Drawing for the job (mm, zero at the part's lowest x, y, z). A direction names the side the tool comes from. Coordinates: 2 decimals unless noted, no trailing zeros. Write each loop counter-clockwise with the first axis right and the second up, starting at its lowest first coordinate (ties: lowest second). Pieces come first, ordered by that corner, then holes. Notation, with made-up numbers: M 53,-9.75 L 58,-9.75 A19 ccw 58,-0.75 Z; hole C 1.5,88 d7. An arc over 180 degrees is marked long. Use a Markdown table: item, result. Add a question column.
Q1. Slice it at C-C on x = 11. Write the cut outline in (y, z), then the cut area to 3 significant figures.
Q2. Slice it at B-B on z = 1.5. Write the cut outline in (x, y).
Q3. Pin check, flat tips, straight feed: pin 1 Ø1.5 at (x, z) = (7, 7.5) entering from -Y; pin 2 Ø4 at (y, z) = (18, 4.5) entering from -X; pin 3 Ø1 at (x, y) = (1.5, 25.5) entering from -Z; pin 4 Ø3 at (x, y) = (8, 43) entering from +Z. Stop position of each tip, or through.
Q4. Wall check: L1, parallel to Y at x = 11.5, z = 4.5; L2, parallel to X at y = 19.5, z = 4.75 (1 decimal); L3, parallel to Z at x = 6.75, y = 6 (1 decimal). Give the ranges that are in metal, low to high. Write a range as from..to.
Q5. Tool access for the marked faces 1 and 2: list every direction of +Z, -Z, +X, -X, +Y, -Y with a clear straight run to the whole face (end or side of a thin tool).
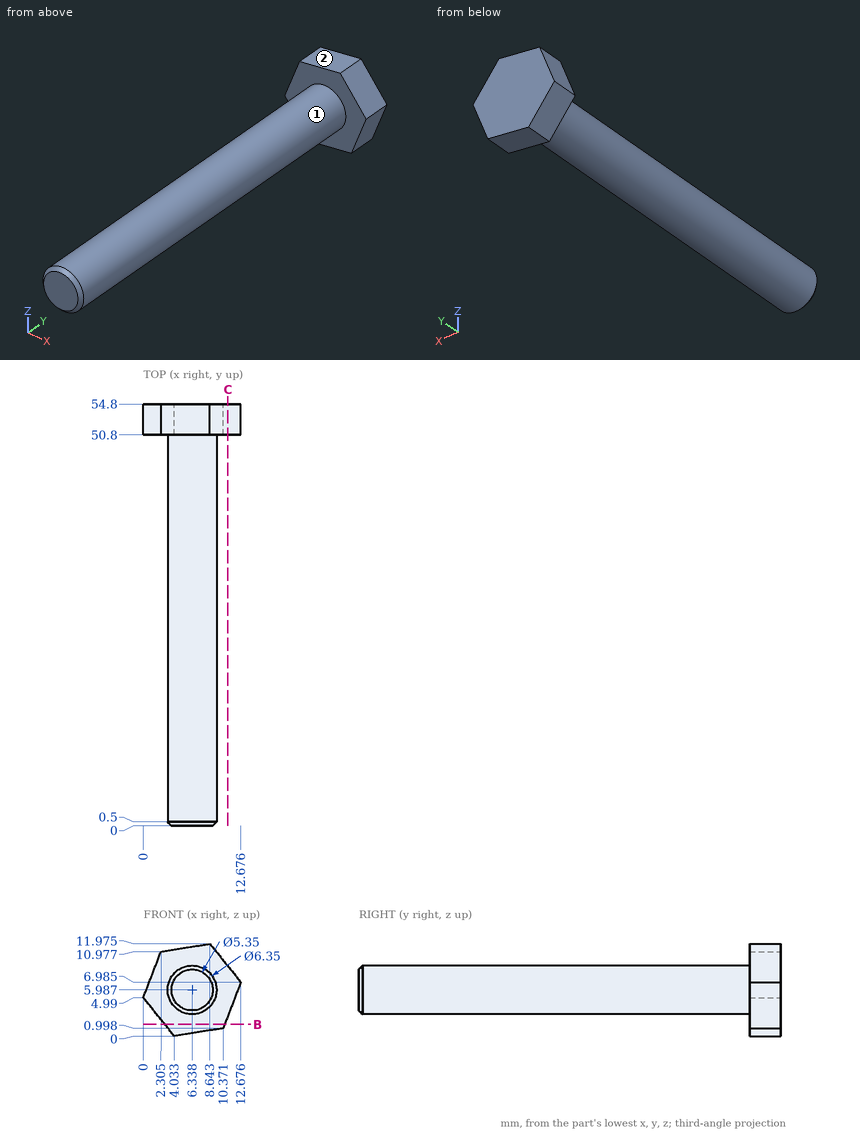
Recorded:
| question | item | result |
|---|---|---|
| 1 | outline | M 50.8,2.63 L 54.8,2.63 L 54.8,9.06 L 50.8,9.06 Z |
| 1 | area | 25.7 mm² |
| 2 | outline | M 2.82,50.8 L 10.56,50.8 L 10.56,54.8 L 2.82,54.8 Z |
| 3 | pin 1 | y = 0 |
| 3 | pin 2 | x = 3.16 |
| 3 | pin 3 | through |
| 3 | pin 4 | z = 9.16 |
| 4 | L1 | 50.8..54.8 |
| 4 | L2 | 3.4..9.3 |
| 4 | L3 | 2.8..9.1 |
| 5 | face 1 | -Y |
| 5 | face 2 | +Z, -X, +Y, -Y |
